from build123d import *

# Parameters (mm, degrees)
SKETCH1_R           = 8
SKETCH1_R_2         = 4
SKETCH1_R_3         = 5
SKETCH1_R_4         = 3.5
BOSS_EXTRUDE1_DEPTH = 21
SKETCH1_4_R         = 8
SKETCH1_4_R_2       = 4
CUT_EXTRUDE1_DEPTH  = 8
SKETCH1_5_R         = 5
SKETCH1_5_R_2       = 3.5
CUT_EXTRUDE2_DEPTH  = 8
CUT_EXTRUDE3_START  = 21
SKETCH1_6_R         = 5
SKETCH1_6_R_2       = 3.5
CUT_EXTRUDE3_DEPTH  = 7
CUT_EXTRUDE4_START  = -14
SKETCH1_7_R         = 5
SKETCH1_7_R_2       = 3.5
CUT_EXTRUDE4_DEPTH  = 7
FILLET2_START       = -8
FILLET2_DEPTH       = 16
FILLET2_START_2     = -22
FILLET2_2_DEPTH     = 8
FILLET2_START_3     = 14
FILLET2_3_DEPTH     = 8
CUT_EXTRUDE5_DEPTH  = 10


with BuildPart() as part:
    # Sketch1 → Boss-Extrude1 (new, symmetric)
    # profile 1 of 4: a face of its own
    with BuildSketch(Plane(origin=(0, 0, 0), x_dir=(0, 0, -1), z_dir=(1, 0, 0))):
        with BuildLine():
            Line((50.3, 4.990991885), (0.48, 7.985587017))
            ThreePointArc((0.48, 7.985587017), (5.824087911, 5.48452368), (8, 0))
            ThreePointArc((8, 0), (5.824087911, -5.48452368), (0.48, -7.985587017))
            Line((0.48, -7.985587017), (50.3, -4.990991885))
            ThreePointArc((50.3, -4.990991885), (45, 0), (50.3, 4.990991885))
        make_face()
    # profile 2 of 4: a face of its own
    with BuildSketch(Plane(origin=(0, 0, 0), x_dir=(0, 0, -1), z_dir=(1, 0, 0))):
        Circle(SKETCH1_R)
        with Locations(Location((0, 0, 0), (0, 0, 180))):
            Circle(SKETCH1_R_2, mode=Mode.SUBTRACT)
    # profile 3 of 4: a face of its own
    with BuildSketch(Plane(origin=(0, 0, 0), x_dir=(0, 0, -1), z_dir=(1, 0, 0))):
        with Locations((50, 0)):
            Circle(SKETCH1_R_3)
        with Locations((50, 0)):
            Circle(SKETCH1_R_4, mode=Mode.SUBTRACT)
    # profile 4 of 4: a face of its own
    with BuildSketch(Plane(origin=(0, 0, 0), x_dir=(0, 0, -1), z_dir=(1, 0, 0))):
        with Locations((50, 0)):
            Circle(SKETCH1_R_4)
    extrude(amount=BOSS_EXTRUDE1_DEPTH, both=True)

    # Sketch1<4> → Cut-Extrude1 (cut, symmetric)
    with BuildSketch(Plane(origin=(0, 0, 0), x_dir=(0, 0, -1), z_dir=(1, 0, 0))):
        Circle(SKETCH1_4_R)
        with Locations(Location((0, 0, 0), (0, 0, 180))):
            Circle(SKETCH1_4_R_2, mode=Mode.SUBTRACT)
    extrude(amount=CUT_EXTRUDE1_DEPTH, both=True, mode=Mode.SUBTRACT)

    # Sketch1<5> → Cut-Extrude2 (cut, symmetric)
    with BuildSketch(Plane(origin=(0, 0, 0), x_dir=(0, 0, -1), z_dir=(1, 0, 0))):
        with Locations((50, 0)):
            Circle(SKETCH1_5_R)
        with Locations((50, 0)):
            Circle(SKETCH1_5_R_2, mode=Mode.SUBTRACT)
    extrude(amount=CUT_EXTRUDE2_DEPTH, both=True, mode=Mode.SUBTRACT)

    # Sketch1<6> → Cut-Extrude3 (cut)
    with BuildSketch(Plane(origin=(0, 0, 0), x_dir=(0, 0, -1), z_dir=(1, 0, 0)).offset(CUT_EXTRUDE3_START)):
        with Locations((50, 0)):
            Circle(SKETCH1_6_R)
        with Locations((50, 0)):
            Circle(SKETCH1_6_R_2, mode=Mode.SUBTRACT)
    extrude(amount=-CUT_EXTRUDE3_DEPTH, mode=Mode.SUBTRACT)

    # Sketch1<7> → Cut-Extrude4 (cut)
    with BuildSketch(Plane(origin=(0, 0, 0), x_dir=(0, 0, -1), z_dir=(1, 0, 0)).offset(CUT_EXTRUDE4_START)):
        with Locations((50, 0)):
            Circle(SKETCH1_7_R)
        with Locations((50, 0)):
            Circle(SKETCH1_7_R_2, mode=Mode.SUBTRACT)
    extrude(amount=-CUT_EXTRUDE4_DEPTH, mode=Mode.SUBTRACT)

    # Fillet2: read off the stored shape, not the designer's step
    # Fillet2 outline → Fillet2 (cut)
    with BuildSketch(Plane.YZ.offset(FILLET2_START)):
        with BuildLine():
            ThreePointArc((-4.990991885, -50.3), (-4.9190545, -49.10395155), (-4.564624299, -47.959361617))
            ThreePointArc((-4.564624299, -47.959361617), (-4.892264664, -48.132066584), (-5.13796127, -47.854923314))
            Line((-5.13796127, -47.854923314), (-4.990991885, -50.3))
        make_face()
        with BuildLine():
            ThreePointArc((5.13796127, -47.854923314), (4.892264664, -48.132066584), (4.564624299, -47.959361617))
            ThreePointArc((4.564624299, -47.959361617), (4.9190545, -49.10395155), (4.990991885, -50.3))
            Line((4.990991885, -50.3), (5.13796127, -47.854923314))
        make_face()
    extrude(amount=FILLET2_DEPTH, mode=Mode.SUBTRACT)

    # Fillet2 2 outline → Fillet2 2 (cut)
    with BuildSketch(Plane.YZ.offset(FILLET2_START_2)):
        with BuildLine():
            ThreePointArc((-4.990991885, -50.3), (-4.9190545, -49.10395155), (-4.564624299, -47.959361617))
            ThreePointArc((-4.564624299, -47.959361617), (-4.892264664, -48.132066584), (-5.13796127, -47.854923314))
            Line((-5.13796127, -47.854923314), (-4.990991885, -50.3))
        make_face()
        with BuildLine():
            ThreePointArc((5.13796127, -47.854923314), (4.892264664, -48.132066584), (4.564624299, -47.959361617))
            ThreePointArc((4.564624299, -47.959361617), (4.9190545, -49.10395155), (4.990991885, -50.3))
            Line((4.990991885, -50.3), (5.13796127, -47.854923314))
        make_face()
    extrude(amount=FILLET2_2_DEPTH, mode=Mode.SUBTRACT)

    # Fillet2 3 outline → Fillet2 3 (cut)
    with BuildSketch(Plane.YZ.offset(FILLET2_START_3)):
        with BuildLine():
            ThreePointArc((-4.990991885, -50.3), (-4.9190545, -49.10395155), (-4.564624299, -47.959361617))
            ThreePointArc((-4.564624299, -47.959361617), (-4.892264664, -48.132066584), (-5.13796127, -47.854923314))
            Line((-5.13796127, -47.854923314), (-4.990991885, -50.3))
        make_face()
        with BuildLine():
            ThreePointArc((5.13796127, -47.854923314), (4.892264664, -48.132066584), (4.564624299, -47.959361617))
            ThreePointArc((4.564624299, -47.959361617), (4.9190545, -49.10395155), (4.990991885, -50.3))
            Line((4.990991885, -50.3), (5.13796127, -47.854923314))
        make_face()
    extrude(amount=FILLET2_3_DEPTH, mode=Mode.SUBTRACT)

    # Sketch3 → Cut-Extrude5 (cut, symmetric)
    with BuildSketch(Plane(origin=(0, 0, 0), x_dir=(1, 0, 0), z_dir=(0, 1, 0))):
        with BuildLine():
            Line((-8, -3.76), (8, -3.76))
            Line((8, -3.76), (8, 5.858563907))
            ThreePointArc((8, 5.858563907), (-0.18107936, 10.23314684), (-8, 5.24))
            Line((-8, 5.24), (-8, -3.76))
        make_face()
    extrude(amount=CUT_EXTRUDE5_DEPTH, both=True, mode=Mode.SUBTRACT)


solid = part.part
Design review of the part built by this model. Coordinates are the model's own, in mm. A direction names the side the tool comes from. Coordinates: 2 decimals unless noted, no trailing zeros. Loops run counter-clockwise (first coordinate to the right, second up) from the corner with the lowest first, then second, coordinate; pieces in that order, holes last. Notation, with made-up numbers: (-7.75, 69.5) -> (45.25, 69.5) arc R24 cw to (45.25, 95.5) -> close; hole circle Ø6 at (63.5, 0.5). An arc over 180 degrees is marked (long way). Use a Markdown table: item, result. Add a question column.
Item 1: Wall thickness on L1, parallel to Z at x = 9.5, y = -0.25; L2, parallel to Y at x = 17.75, z = 0; L3, parallel to X at y = -4.5, z = 1: over which ranges is each line inside the solid? List them lowest first. Write a range as from..to.
Item 2: We need section D-D, the plane z = -26. Write out the cut boundary in (x, y), and give its area (3 significant figures).
Item 3: We need section B-B, the plane y = 0. Count the separate pieces of the cut face and the enclosed holes in it, and give its area (3 significant figures).
Item 4: Machinability: for faces 4 (the flat face through (-8, -3.5, -51.04)), 5 (the cylindrical face through (17.549, 0.154, -46.503)), 6 (the cylindrical face through (-7, 0, -8)), 7 (the cylindrical face through (-17.451, 0.154, -46.503)), which of the approach directions +Z, -Z, +X, -X, +Y, -Y give a long, thin tool a straight path to every point of the face, cutting with its end or side? Answer none if there is none.
Item 5: We need section A-A, the plane x = 16. Write out the cut boundary in (y, z), and give its area (3 significant figures).
Item 6: The part is to be moulded in two halves that separate along Z. For faces 1 (the flat face through (8, -3.5, -51.04)), 2 (the flat face through (21, 0, -20)), 3 (the cylindrical face through (-11, 0, -55)), say which applies: +Z half, -Z half, draft (parallel to the pull), parting line (faces both ways), or undercut.
Item 7: Clearance check with flat-ended pins moving along their axes: P1, Ø12, axis at x = 15, z = -46, coming from the +Y side; P2, Ø5, axis at x = -16, z = -14, coming from the +Y side; P3, Ø1, axis at x = -16, z = -29, coming from the +Y side. State where each tip first meets the part, or that it passes through.
Item 8: We need section C-C, the plane x = -1. Write out the cut boundary in (y, z).
Numbers:
| question | item | result |
|---|---|---|
| 1 | L1 | z = -54.99..-3.99, 3.99..8 |
| 1 | L2 | y = -8..-4, 4..8 |
| 1 | L3 | x = -21..-8, 8..21 |
| 2 | outline | (-21, -6.45) -> (21, -6.45) -> (21, 6.45) -> (-21, 6.45) -> close |
| 2 | area | 542 mm^2 |
| 3 | separate pieces | 3 |
| 3 | enclosed holes | 1 |
| 3 | area | 2,070 mm^2 |
| 4 | face 4 | none |
| 4 | face 5 | +X |
| 4 | face 6 | +Z |
| 4 | face 7 | -X |
| 5 | outline | (-7.99, -0.48) -> (-5.14, -47.85) arc R0.3 ccw to (-4.56, -47.96) arc R5 cw to (4.56, -47.96) arc R0.3 ccw to (5.14, -47.85) -> (7.99, -0.48) arc R8 ccw (long way) to start; circle Ø7 at (0, -50); hole circle Ø8 at (0, 0) |
| 5 | area | 700 mm^2 |
| 6 | face 1 | undercut |
| 6 | face 2 | draft |
| 6 | face 3 | -Z half |
| 7 | P1 | stops at y = 5.61 |
| 7 | P2 | stops at y = 7.32 |
| 7 | P3 | stops at y = 6.3 |
| 8 | outline | (-7.4, -10.16) -> (-5.14, -47.85) arc R0.3 ccw to (-4.56, -47.96) arc R5 cw to (4.56, -47.96) arc R0.3 ccw to (5.14, -47.85) -> (7.4, -10.16) -> close; circle Ø7 at (0, -50) |
